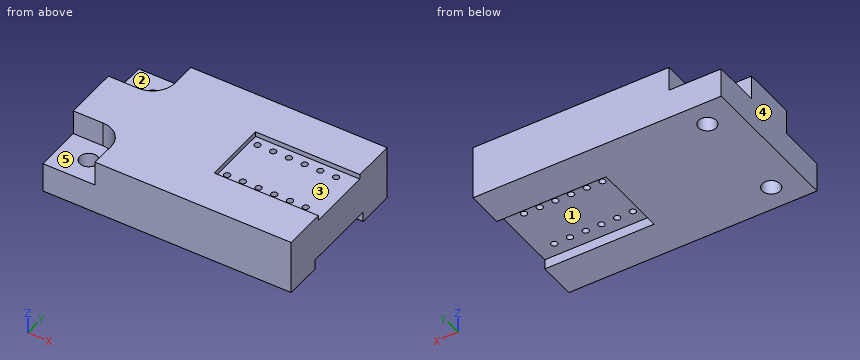
from build123d import *

# Parameters (mm, degrees)
SKIZZE1_W                       = 100
SKIZZE1_H                       = 60
AUFSATZ_LINEAR_AUSTRAGEN1_DEPTH = 12
SKIZZE3_R                       = 3.6
SCHNITT_LINEAR_AUSTRAGEN2_DEPTH = 20
AUFSATZ_LINEAR_AUSTRAGEN2_DEPTH = 10
SKIZZE9_W                       = 42
SKIZZE9_H                       = 26
SCHNITT_LINEAR_AUSTRAGEN6_DEPTH = 2
SKIZZE10_W                      = 44
SKIZZE10_H                      = 30
SCHNITT_LINEAR_AUSTRAGEN7_DEPTH = 4
SKIZZE11_R                      = 1.25
SCHNITT_LINEAR_AUSTRAGEN8_DEPTH = 119.321595662


with BuildPart() as part:
    # Skizze1 → Aufsatz-Linear austragen1 (new body)
    with BuildSketch(Plane.XY):
        with Locations((-50, -30)):
            Rectangle(SKIZZE1_W, SKIZZE1_H)
    extrude(amount=AUFSATZ_LINEAR_AUSTRAGEN1_DEPTH)

    # Skizze3 → Schnitt-Linear austragen2 (cut)
    with BuildSketch(Plane.XY.offset(12)):
        with Locations((-88, -10)):
            Circle(SKIZZE3_R)
        with Locations((-88, -50)):
            Circle(SKIZZE3_R)
    extrude(amount=-SCHNITT_LINEAR_AUSTRAGEN2_DEPTH, mode=Mode.SUBTRACT)

    # Skizze5 → Aufsatz-Linear austragen2 (add)
    with BuildSketch(Plane.XY.offset(12)):
        with BuildLine():
            Line((-100, -41), (-88, -41))
            ThreePointArc((-88, -41), (-81.636038969, -43.636038969), (-79, -50))
            Line((-79, -50), (-79, -60))
            Line((-79, -60), (0, -60))
            Line((0, -60), (0, 0))
            Line((0, 0), (-79, 0))
            Line((-79, 0), (-79, -10))
            ThreePointArc((-79, -10), (-81.636038969, -16.363961031), (-88, -19))
            Line((-88, -19), (-100, -19))
            Line((-100, -19), (-100, -41))
        make_face()
    extrude(amount=AUFSATZ_LINEAR_AUSTRAGEN2_DEPTH)

    # Skizze9 → Schnitt-Linear austragen6 (cut)
    with BuildSketch(Plane.XY.offset(22)):
        with Locations((-21, -30)):
            Rectangle(SKIZZE9_W, SKIZZE9_H)
    extrude(amount=-SCHNITT_LINEAR_AUSTRAGEN6_DEPTH, mode=Mode.SUBTRACT)

    # Skizze10 → Schnitt-Linear austragen7 (cut)
    with BuildSketch(Plane(origin=(0, 0, 0), x_dir=(-1, 0, 0), z_dir=(0, 0, -1))):
        with Locations((22, -30)):
            Rectangle(SKIZZE10_W, SKIZZE10_H)
    extrude(amount=-SCHNITT_LINEAR_AUSTRAGEN7_DEPTH, mode=Mode.SUBTRACT)

    # Skizze11 → Schnitt-Linear austragen8 (cut, through all)
    with BuildSketch(Plane.XY.offset(20)):
        with Locations((-39, -20.5)):
            Circle(SKIZZE11_R)
        with Locations((-39, -39.5)):
            Circle(SKIZZE11_R)
        with Locations((-32.667, -20.5)):
            Circle(SKIZZE11_R)
        with Locations((-32.667, -39.5)):
            Circle(SKIZZE11_R)
        with Locations((-26.334, -20.5)):
            Circle(SKIZZE11_R)
        with Locations((-26.334, -39.5)):
            Circle(SKIZZE11_R)
        with Locations((-20.001, -20.5)):
            Circle(SKIZZE11_R)
        with Locations((-20.001, -39.5)):
            Circle(SKIZZE11_R)
        with Locations((-13.668, -20.5)):
            Circle(SKIZZE11_R)
        with Locations((-13.668, -39.5)):
            Circle(SKIZZE11_R)
        with Locations((-7.335, -20.5)):
            Circle(SKIZZE11_R)
        with Locations((-7.335, -39.5)):
            Circle(SKIZZE11_R)
    extrude(amount=-SCHNITT_LINEAR_AUSTRAGEN8_DEPTH, mode=Mode.SUBTRACT)


solid = part.part
Part model, mm, in its own coordinate system. Face numbers are marked on the shaded views. A direction names the side the tool comes from. Coordinates: 2 decimals unless noted, no trailing zeros. Loops run counter-clockwise (first coordinate to the right, second up) from the corner with the lowest first, then second, coordinate; pieces in that order, holes last. Notation, with made-up numbers: M -3.5,68.5 L 33.5,68.5 A16 ccw 33.5,98.5 Z; hole C 89.5,23.5 d8. An arc over 180 degrees is marked long. Use a Markdown table: item, result. Add a question column.
Q1. Pin check, flat tips, straight feed: P1, Ø5, axis at x = -14.5, y = -30, coming from the -Z side; P2, Ø1.2, axis at y = -31, z = 2.5, coming from the +X side; P3, Ø5, axis at y = -3.5, z = 18.5, coming from the -X side. Stop position of each tip, or through.
Q2. Cut at B-B (y = -39.5). Give the number of separate pieces and of enclosed holes in the cut face, and give its area (3 significant figures).
Q3. Cut at A-A (x = -39). Write the cut outline in (y, z).
Q4. Which spindle directions (+Z, -Z, +X, -X, +Y, -Y) get a long thin tool onto all of the face, cutting with end or side? Do the marked faces 1, 2, 3, 4 and 5. Say none if no direction does.
Q5. Probe L1, parallel to Y at x = -13.5, z = 5.5; L2, parallel to Y at x = -88, z = 8.5; L3, parallel to Y at x = -9.5, z = 21. List the from-to ranges inside material, lowest first.
Q6. Cut at C-C (z = 2). Write the cut outline in (x, y).
Worked out:
| question | item | result |
|---|---|---|
| 1 | P1 | stops at z = 4 |
| 1 | P2 | stops at x = -44 |
| 1 | P3 | stops at x = -79 |
| 2 | separate pieces | 7 |
| 2 | enclosed holes | 0 |
| 2 | area | 1,700 mm2 |
| 3 | outline | M -60,0 L -45,0 L -45,4 L -40.75,4 L -40.75,20 L -43,20 L -43,22 L -60,22 Z; M -38.25,4 L -21.75,4 L -21.75,20 L -38.25,20 Z; M -19.25,4 L -15,4 L -15,0 L 0,0 L 0,22 L -17,22 L -17,20 L -19.25,20 Z |
| 4 | face 1 | -Z, +X |
| 4 | face 2 | +Z, -X, +Y |
| 4 | face 3 | +Z, +X |
| 4 | face 4 | +Z, -Z, -X, +Y, -Y |
| 4 | face 5 | +Z, -X, -Y |
| 5 | L1 | y = -60 to -40.74, -38.26 to -21.74, -19.26 to 0 |
| 5 | L2 | y = -60 to -53.6, -46.4 to -13.6, -6.4 to 0 |
| 5 | L3 | y = -60 to -43, -17 to 0 |
| 6 | outline | M -100,-60 L 0,-60 L 0,-45 L -44,-45 L -44,-15 L 0,-15 L 0,0 L -100,0 Z; hole C -88,-50 d7.2; hole C -88,-10 d7.2 |
